Check sheet for the modelled part. Datum: model origin and axes. Units: mm. Face numbers are marked on the shaded views. A direction names the side the tool comes from. Give positions to 0.01 mm unless a question says otherwise; leave off trailing zeros. Write each loop counter-clockwise with the first axis right and the second up, starting at its lowest first coordinate (ties: lowest second). Pieces come first, ordered by that corner, then holes. Notation, with made-up numbers: (-10.75, 61.5) -> (-1.75, 61.5) arc R22 cw to (-1.75, 91.5) -> close; hole circle Ø8 at (69.25, 1.25). An arc over 180 degrees is marked (long way). Write each question's results on one line, items separated by ' | '. Start each with the question number.
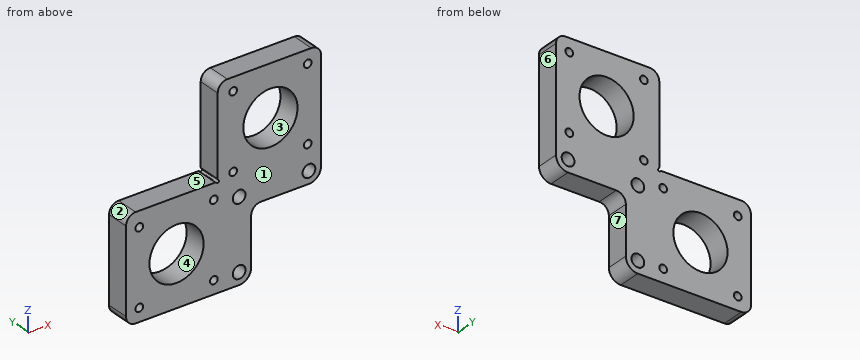
```python
from build123d import *

# Parameters (mm, degrees)
BOSS_EXTRUDE1_DEPTH          = 9.525
F_22_5_22_5_DIAMETER_HOLE1_D = 22.5
M3_CLEARANCE_HOLE1_D         = 3.2
M5_CLEARANCE_HOLE1_D         = 5.3
BOSS_EXTRUDE2_DEPTH          = 9.525
SKETCH17_R                   = 0.5
CUT_EXTRUDE1_DEPTH           = 9.525
FILLET2_R                    = 4
FILLET3_R                    = 5
FILLET4_R                    = 1


with BuildPart() as part:
    # Sketch1 → Boss-Extrude1 (new body)
    with BuildSketch(Plane(origin=(0, 0, 0), x_dir=(1, 0, 0), z_dir=(0, 1, 0))):
        Polygon((60, -21), (60, 31), (31, 31), (31, 60), (-21, 60), (-21, 18), (18, 18), (18, -21), align=None)
    extrude(amount=BOSS_EXTRUDE1_DEPTH)

    # Ø22.5 (22.5) Diameter Hole1 (through all)
    with Locations(Plane(origin=(0, 9.525, 0), x_dir=(1, 0, 0), z_dir=(0, 1, 0))):
        with Locations((0, 39), (39, 0)):
            Hole(F_22_5_22_5_DIAMETER_HOLE1_D / 2)

    # M3 Clearance Hole1 (through all)
    with Locations(Plane(origin=(0, 0, 0), x_dir=(-1, 0, 0), z_dir=(0, -1, 0))):
        with Locations((-54.5, 15.5), (-23.5, 15.5), (-23.5, -15.5), (-54.5, -15.5), (-15.5, 54.5), (-15.5, 23.5), (15.5, 23.5), (15.5, 54.5)):
            Hole(M3_CLEARANCE_HOLE1_D / 2)

    # M5 Clearance Hole1 (through all)
    with Locations(Plane(origin=(0, 9.525, 0), x_dir=(1, 0, 0), z_dir=(0, 1, 0))):
        with Locations((26, 55), (26, 26), (55, 26)):
            Hole(M5_CLEARANCE_HOLE1_D / 2)

    # Sketch16 → Boss-Extrude2 (add)
    with BuildSketch(Plane(origin=(0, 9.525, 0), x_dir=(1, 0, 0), z_dir=(0, 1, 0))):
        Polygon((17.1, 17.1), (-21, 17.1), (-21, 18), (18, 18), (18, -21), (17.1, -21), align=None)
    extrude(amount=-BOSS_EXTRUDE2_DEPTH)

    # Sketch17 → Cut-Extrude1 (cut)
    with BuildSketch(Plane(origin=(0, 9.525, 0), x_dir=(1, 0, 0), z_dir=(0, 1, 0))):
        with Locations((17.1, 17.1)):
            Circle(SKETCH17_R)
    extrude(amount=-CUT_EXTRUDE1_DEPTH, mode=Mode.SUBTRACT)

    # Fillet2
    fillet2_edges = [part.edges().sort_by_distance(p)[0] for p in [
        (17.1, 4.7625, 21),
        (-21, 4.7625, -17.1),
        (-21, 4.7625, -60),
        (31, 4.7625, -31),
        (60, 4.7625, 21),
    ]]
    fillet(fillet2_edges, radius=FILLET2_R)

    # Fillet3
    fillet3_edges = [part.edges().sort_by_distance(p)[0] for p in [
        (31, 4.7625, -60),
        (60, 4.7625, -31),
    ]]
    fillet(fillet3_edges, radius=FILLET3_R)

    # Fillet4
    fillet4_edges = [part.edges().sort_by_distance(p)[0] for p in [
        (16.6, 4.7625, -17.1),
        (17.1, 4.7625, -16.6),
    ]]
    fillet(fillet4_edges, radius=FILLET4_R)


solid = part.part
```
Item 1: Section check B-B on z = 15.5. Record the boundary of the cut face in (x, y) (3 decimals).
Item 2: Section check D-D on y = 3. Count the separate pieces of the cut face and the enclosed holes in it, then the cut area to 3 significant figures.
Item 3: Depth check by flat-ended pin: pin 1 Ø3 at (y, z) = (3, 0.5) entering from -X; pin 2 Ø1.9 at (x, z) = (54.5, -15.5) entering from +Y; pin 3 Ø1.5 at (x, y) = (11, 3.5) entering from +Z; pin 4 Ø6 at (x, z) = (26, -26) entering from -Y. Enter the tip coordinate at first touch or a pass-through.
Item 4: Section check A-A on x = 39. Record the boundary of the cut face in (y, z) (3 decimals).
Item 5: Mould release check, pull along X, two halves, no side actions. Record for the marked faces 1, 2, 3 and 4: pulls with the +X half, pulls with the -X half, needs draft (parallel to the pull), parting line crosses it, or undercut.
Item 6: Thickness scan on probe 1 along Z at (x, y) = (26, 4); probe 2 along X at (y, z) = (7.75, -26); probe 3 along X at (y, z) = (5.5, -54.5). Record the ranges inside material, lowest first. Write a range as from..to.
Item 7: Set-up check for the marked faces 5, 6 and 7: record each of +Z, -Z, +X, -X, +Y, -Y from which the full face is reachable in a straight line by a thin tool's end or side.
Item 8: Section check C-C on x = -15.5. Record the boundary of the cut face in (y, z) (3 decimals).
Check sheet entries:
1) outline: (17.1, 0) -> (21.9, 0) -> (21.9, 9.525) -> (17.1, 9.525) -> close; (25.1, 0) -> (52.9, 0) -> (52.9, 9.525) -> (25.1, 9.525) -> close; (56.1, 0) -> (60, 0) -> (60, 9.525) -> (56.1, 9.525) -> close
2) separate pieces: 1 | enclosed holes: 13 | area: 3,320 mm^2
3) pin 1: stops at x = 17.1 | pin 2: passes through | pin 3: stops at z = -17.1 | pin 4: stops at y = 0
4) outline: (0, -31) -> (9.525, -31) -> (9.525, -11.25) -> (0, -11.25) -> close; (0, 11.25) -> (9.525, 11.25) -> (9.525, 21) -> (0, 21) -> close
5) face 1: needs draft | face 2: pulls with the -X half | face 3: undercut | face 4: undercut
6) probe 1: z = -60..-57.65, -52.35..-28.65, -23.35..21 | probe 2: x = -21..23.35, 28.65..52.35, 57.65..60 | probe 3: x = -21..-17.1, -13.9..13.9, 17.1..23.4, 28.6..31
7) face 5: +Z, -X, +Y, -Y | face 6: +Z, -Z, +X, +Y, -Y | face 7: -Z, +X, +Y, -Y
8) outline: (0, -60) -> (9.525, -60) -> (9.525, -56.1) -> (0, -56.1) -> close; (0, -52.9) -> (9.525, -52.9) -> (9.525, -25.1) -> (0, -25.1) -> close; (0, -21.9) -> (9.525, -21.9) -> (9.525, -17.1) -> (0, -17.1) -> close
